Source: CAD feature listing. Evaluate the final solid. Frame: model axes, mm. A direction names the side the tool comes from. Coordinates: 2 decimals unless noted, no trailing zeros. Order: outer loops, then holes, each group sorted by start corner. A loop starts at its lowest first (then second) coordinate and runs counter-clockwise, first axis right, second up.
```python
from build123d import *

# Parameters (mm, degrees)
ESQUISSE2_R             = 2.25
ENL_V_MAT_EXTRU_1_DEPTH = 3


with BuildPart() as part:
    # Esquisse1 → Révolution1 (revolve)
    with BuildSketch(Plane.XY, mode=Mode.PRIVATE) as r_volution1_sk:
        Polygon((1.35, 0), (1.35, 8), (4.75, 8), (4.75, 6), (5.25, 6), (5.25, 0), align=None)
    revolve(r_volution1_sk.sketch.rotate(Axis((0, 0, 0), (0, 1, 0)), 90), axis=Axis((0, 0, 0), (0, 1, 0)))

    # Esquisse2 → Enlèv. mat.-Extru.1 (cut)
    with BuildSketch(Plane(origin=(0, 8, 0), x_dir=(1, 0, 0), z_dir=(0, 1, 0))):
        with Locations(Location((0, 0, 0), (0, 0, 270))):
            Circle(ESQUISSE2_R)
    extrude(amount=-ENL_V_MAT_EXTRU_1_DEPTH, mode=Mode.SUBTRACT)


solid = part.part
```
Q1. Section query A-A on x = 0. Output: boundary loops of the cut face in (y, z).
Solutions:
outline: (0, -5.25) - (6, -5.25) - (6, -4.75) - (8, -4.75) - (8, -2.25) - (5, -2.25) - (5, -1.35) - (0, -1.35) - close; (0, 1.35) - (5, 1.35) - (5, 2.25) - (8, 2.25) - (8, 4.75) - (6, 4.75) - (6, 5.25) - (0, 5.25) - close
Q2. Material intervals for line 1 along X through (y, z) = (3, 0); line 2 along X through (y, z) = (5.9, 0); line 3 along Z through (x, y) = (-0.5, 5.5), sorted ascending.
Solutions:
line 1: x = -5.25 to -1.35, 1.35 to 5.25
line 2: x = -5.25 to -2.25, 2.25 to 5.25
line 3: z = -5.23 to -2.19, 2.19 to 5.23
Q3. Section query D-D on x = -3.5. Output: boundary loops of the cut face in (y, z), plus the area to 3 significant figures.
Solutions:
outline: (0, -3.91) - (6, -3.91) - (6, -3.21) - (8, -3.21) - (8, 3.21) - (6, 3.21) - (6, 3.91) - (0, 3.91) - close
area: 59.8 mm2
Q4. Pull-direction query (X, two-part tool) for faces 1 (the cylindrical face through (0.676, 6.521, 2.146)), 2 (the flat face through (-1.5, 5, 0.5)), 3 (the cylindrical face through (4.637, 6.986, 1.03)), 4 (the flat face through (1, 8, -2.2)); classes: pulls with the +X half, pulls with the -X half, needs draft (parallel to the pull), parting line crosses it, or undercut.
Solutions:
face 1: undercut
face 2: undercut
face 3: parting line crosses it
face 4: needs draft
Q5. Pin query (flat end, axial travel): P1, Ø3.5, axis at x = 0, z = 0, coming from the +Y side; P2, Ø1, axis at x = -2.5, y = 6, coming from the -Z side; P3, Ø1.5, axis at x = -3, y = 5, coming from the -Z side. Return the tip coordinate at first contact, or that it passes through.
Solutions:
P1: stops at y = 5
P2: stops at z = -4.85
P3: stops at z = -4.74
Q6. Section query C-C on y = 4.5. Output: boundary loops of the cut face in (x, z), plus the area to 3 significant figures.
Solutions:
outline: circle Ø10.5 at (0, 0); hole circle Ø2.7 at (0, 0)
area: 80.9 mm2
Q7. Set-up query: faces 5 (the cylindrical face through (0.82, 2.54, 1.07)), 6 (the flat face through (3, 6, -4)). Return all of +Z, -Z, +X, -X, +Y, -Y with unobstructed straight access to the full face (end or side cutting, diameter ignored); none if empty.
Solutions:
face 5: +Y, -Y
face 6: +Y
Q8. Section query B-B on z = 0. Output: boundary loops of the cut face in (x, y).
Solutions:
outline: (-5.25, 0) - (-1.35, 0) - (-1.35, 5) - (-2.25, 5) - (-2.25, 8) - (-4.75, 8) - (-4.75, 6) - (-5.25, 6) - close; (1.35, 0) - (5.25, 0) - (5.25, 6) - (4.75, 6) - (4.75, 8) - (2.25, 8) - (2.25, 5) - (1.35, 5) - close
